from build123d import *

# Parameters (mm, degrees)
SKETCH1_R           = 2.975
BOSS_EXTRUDE1_DEPTH = 3.175


with BuildPart() as part:
    # Sketch1 → Boss-Extrude1 (new body)
    with BuildSketch(Plane(origin=(0, 0, 0), x_dir=(1, 0, 0), z_dir=(0, 1, 0))):
        with BuildLine():
            ThreePointArc((11.882947492, 0.263140878), (12.316055042, 0.553383075), (12.455331476, 1.055801982))
            ThreePointArc((12.455331476, 1.055801982), (12.372768024, 1.778935478), (12.248256827, 2.4960378))
            ThreePointArc((12.248256827, 2.4960378), (11.973074304, 2.938866505), (11.475739976, 3.095331356))
            ThreePointArc((11.475739976, 3.095331356), (9.460172752, 4.320316135), (9.854306858, 6.645774639))
            ThreePointArc((9.854306858, 6.645774639), (10.061743337, 7.124097533), (9.90728196, 7.622057738))
            ThreePointArc((9.90728196, 7.622057738), (9.446869679, 8.185759174), (8.95442941, 8.721708201))
            ThreePointArc((8.95442941, 8.721708201), (8.483519867, 8.945464509), (7.980544323, 8.80821188))
            ThreePointArc((7.980544323, 8.80821188), (5.622664502, 8.749036741), (4.696993425, 10.918421909))
            ThreePointArc((4.696993425, 10.918421909), (4.612899215, 11.43296136), (4.213740424, 11.768364017))
            ThreePointArc((4.213740424, 11.768364017), (3.521656961, 11.99366217), (2.817633925, 12.178297872))
            ThreePointArc((2.817633925, 12.178297872), (2.300507814, 12.111940737), (1.951582234, 11.724547368))
            ThreePointArc((1.951582234, 11.724547368), (0, 10.4), (-1.951582234, 11.724547368))
            ThreePointArc((-1.951582234, 11.724547368), (-2.300507814, 12.111940737), (-2.817633925, 12.178297872))
            ThreePointArc((-2.817633925, 12.178297872), (-3.521656961, 11.99366217), (-4.213740424, 11.768364017))
            ThreePointArc((-4.213740424, 11.768364017), (-4.612899215, 11.43296136), (-4.696993425, 10.918421909))
            ThreePointArc((-4.696993425, 10.918421909), (-5.622664502, 8.749036741), (-7.980544323, 8.80821188))
            ThreePointArc((-7.980544323, 8.80821188), (-8.483519867, 8.945464509), (-8.95442941, 8.721708201))
            ThreePointArc((-8.95442941, 8.721708201), (-9.446869679, 8.185759174), (-9.90728196, 7.622057738))
            ThreePointArc((-9.90728196, 7.622057738), (-10.061743337, 7.124097533), (-9.854306858, 6.645774639))
            ThreePointArc((-9.854306858, 6.645774639), (-9.460172752, 4.320316135), (-11.475739976, 3.095331356))
            ThreePointArc((-11.475739976, 3.095331356), (-11.973074304, 2.938866505), (-12.248256827, 2.4960378))
            ThreePointArc((-12.248256827, 2.4960378), (-12.372768024, 1.778935478), (-12.455331476, 1.055801982))
            ThreePointArc((-12.455331476, 1.055801982), (-12.316055042, 0.553383075), (-11.882947492, 0.263140878))
            ThreePointArc((-11.882947492, 0.263140878), (-10.294142996, -1.480074318), (-11.327469272, -3.600295003))
            ThreePointArc((-11.327469272, -3.600295003), (-11.661262247, -4.000800849), (-11.653349243, -4.522106966))
            ThreePointArc((-11.653349243, -4.522106966), (-11.370399942, -5.192687663), (-11.048901253, -5.845663444))
            ThreePointArc((-11.048901253, -5.845663444), (-10.660106293, -6.193026599), (-10.138836257, -6.203038252))
            ThreePointArc((-10.138836257, -6.203038252), (-7.859795573, -6.810551633), (-7.582807109, -9.152853138))
            ThreePointArc((-7.582807109, -9.152853138), (-7.647081821, -9.670242202), (-7.358585614, -10.104514722))
            ThreePointArc((-7.358585614, -10.104514722), (-6.758010218, -10.51566916), (-6.13452295, -10.891172029))
            ThreePointArc((-6.13452295, -10.891172029), (-5.619649116, -10.973194086), (-5.175716149, -10.699796566))
            ThreePointArc((-5.175716149, -10.699796566), (-2.930018591, -9.978726926), (-1.430657267, -11.799445071))
            ThreePointArc((-1.430657267, -11.799445071), (-1.205006949, -12.269449983), (-0.727523045, -12.478810449))
            ThreePointArc((-0.727523045, -12.478810449), (0, -12.5), (0.727523045, -12.478810449))
            ThreePointArc((0.727523045, -12.478810449), (1.205006949, -12.269449983), (1.430657267, -11.799445071))
            ThreePointArc((1.430657267, -11.799445071), (2.930018591, -9.978726926), (5.175716149, -10.699796566))
            ThreePointArc((5.175716149, -10.699796566), (5.619649116, -10.973194086), (6.13452295, -10.891172029))
            ThreePointArc((6.13452295, -10.891172029), (6.758010218, -10.51566916), (7.358585614, -10.104514722))
            ThreePointArc((7.358585614, -10.104514722), (7.647081821, -9.670242202), (7.582807109, -9.152853138))
            ThreePointArc((7.582807109, -9.152853138), (7.859795573, -6.810551633), (10.138836257, -6.203038252))
            ThreePointArc((10.138836257, -6.203038252), (10.660106293, -6.193026599), (11.048901253, -5.845663444))
            ThreePointArc((11.048901253, -5.845663444), (11.370399942, -5.192687663), (11.653349243, -4.522106966))
            ThreePointArc((11.653349243, -4.522106966), (11.661262247, -4.000800849), (11.327469272, -3.600295003))
            ThreePointArc((11.327469272, -3.600295003), (10.294142996, -1.480074318), (11.882947492, 0.263140878))
        make_face()
        Circle(SKETCH1_R, mode=Mode.SUBTRACT)
    extrude(amount=BOSS_EXTRUDE1_DEPTH)


solid = part.part
Verification items for the finished model (mm, model axes). Give positions to 0.01 mm unless a question says otherwise; leave off trailing zeros. Loops run counter-clockwise (first coordinate to the right, second up) from the corner with the lowest first, then second, coordinate; pieces in that order, holes last.
1) Thickness scan on line 1 along X through (y, z) = (1.05, 10.25); line 2 along Z through (x, y) = (0.75, 2.3); line 3 along X through (y, z) = (1.9, 0) (3 decimals). Record the ranges inside material, lowest first.
2) Sectioned sample at D-D, the plane z = -9.75. Enter the section's corners in (x, y) (3 decimals).
3) Depth check by flat-ended pin: pin 1 Ø1.5 at (x, y) = (-6.5, 2.5) entering from +Z. Enter the tip coordinate at first touch or a pass-through.
4) Sectioned sample at C-C, the plane z = 7.25. Enter the section's corners in (x, y) (3 decimals), then the cut area to 3 significant figures.
5) Sectioned sample at B-B, the plane z = 0.75. Enter the section's corners in (x, y) (3 decimals).
6) Draft check along X on faces 1 (the cylindrical face through (-5.59, 1.57, -8.77)), 2 (the cylindrical face through (-12.37, 1.57, -1.79)), 3 (the cylindrical face through (0, 1.6, 12.5)), 4 (the cylindrical face through (-7.883, 1.565, 6.784)). Enter one of: pulls with the +X half, pulls with the -X half, needs draft (parallel to the pull), parting line crosses it, or undercut.
7) Sectioned sample at A-A, the plane x = 0. Enter the section's corners in (y, z) (3 decimals), then the cut area to 3 significant figures.
Answers:
1. line 1: x = -7.15 to -4.69, -2.35 to 2.35, 4.69 to 7.15
1. line 2: z = -10.54 to -2.88, 2.88 to 12.48
1. line 3: x = -11.257 to -2.975, 2.975 to 11.257
2. outline: (-4.803, 0) - (4.803, 0) - (4.803, 3.175) - (-4.803, 3.175) - close
3. pin 1: stops at z = 10.99
4. outline: (-7.567, 0) - (7.567, 0) - (7.567, 3.175) - (-7.567, 3.175) - close
4. area: 48.0 mm2
5. outline: (-10.542, 0) - (-2.879, 0) - (-2.879, 3.175) - (-10.542, 3.175) - close; (2.879, 0) - (10.542, 0) - (10.542, 3.175) - (2.879, 3.175) - close
6. face 1: undercut
6. face 2: pulls with the -X half
6. face 3: parting line crosses it
6. face 4: undercut
7. outline: (0, -10.4) - (3.175, -10.4) - (3.175, -2.975) - (0, -2.975) - close; (0, 2.975) - (3.175, 2.975) - (3.175, 12.5) - (0, 12.5) - close
7. area: 53.8 mm2
